```python
from build123d import *

# Parameters (mm, degrees)
SZKIC1_R                    = 4.5
SZKIC1_R_2                  = 6.5
DODANIE_WYCI_GNI_CIE1_DEPTH = 10


with BuildPart() as part:
    # Szkic1 → Dodanie-wyciągnięcie1 (new body)
    with BuildSketch(Plane(origin=(0, 0, 0), x_dir=(1, 0, 0), z_dir=(0, 1, 0))):
        with BuildLine():
            Line((-1.5, 30.463092423), (-1.5, 29.063092423))
            ThreePointArc((-1.5, 29.063092423), (0, 27.563092423), (1.5, 29.063092423))
            Line((1.5, 29.063092423), (1.5, 30.463092423))
            ThreePointArc((1.5, 30.463092423), (0, -30.5), (-1.5, 30.463092423))
        make_face()
        with Locations(Location((0, 0, 0), (0, 0, 270))):
            Circle(SZKIC1_R, mode=Mode.SUBTRACT)
        with Locations(Location((0, 17.5, 0), (0, 0, 270))):
            Circle(SZKIC1_R_2, mode=Mode.SUBTRACT)
        with Locations(Location((13.682050943, 10.911071533, 0), (0, 0, 270))):
            Circle(SZKIC1_R_2, mode=Mode.SUBTRACT)
        with Locations(Location((17.061238463, -3.894116344, 0), (0, 0, 270))):
            Circle(SZKIC1_R_2, mode=Mode.SUBTRACT)
        with Locations(Location((7.592965435, -15.766955188, 0), (0, 0, 270))):
            Circle(SZKIC1_R_2, mode=Mode.SUBTRACT)
        with Locations(Location((-7.592965435, -15.766955188, 0), (0, 0, 270))):
            Circle(SZKIC1_R_2, mode=Mode.SUBTRACT)
        with Locations(Location((-17.061238463, -3.894116344, 0), (0, 0, 270))):
            Circle(SZKIC1_R_2, mode=Mode.SUBTRACT)
        with Locations(Location((-13.682050943, 10.911071533, 0), (0, 0, 270))):
            Circle(SZKIC1_R_2, mode=Mode.SUBTRACT)
    extrude(amount=DODANIE_WYCI_GNI_CIE1_DEPTH)


solid = part.part
```
Design review of the part built by this model. Coordinates are the model's own, in mm. A direction names the side the tool comes from. Give positions to 0.01 mm unless a question says otherwise; leave off trailing zeros. Write each loop counter-clockwise with the first axis right and the second up, starting at its lowest first coordinate (ties: lowest second). Pieces come first, ordered by that corner, then holes.
(1) Mouldability with a two-part tool opening along X and no side actions: class faces 3 (the face through (-6, 10, 0)), 4 (the face through (-13.396, 4.93, -17.405)), 5 (the face through (1.32, 4.93, 30.47)), 6 (the face through (-0.033, 4.93, -27.563)) as +X half, -X half, draft (parallel to the pull), parting line (faces both ways), or undercut.
Checked values:
face 3: draft
face 4: undercut
face 5: parting line
face 6: undercut
(2) Add section A-A (x = 0). Give the boundary of the cut face in (y, z).
Checked values:
outline: (0, -27.56) - (10, -27.56) - (10, -24) - (0, -24) - close; (0, -11) - (10, -11) - (10, -4.5) - (0, -4.5) - close; (0, 4.5) - (10, 4.5) - (10, 30.5) - (0, 30.5) - close
(3) Tool access review of faces 1 (the face through (13.106, 4.93, -1.264)), 2 (the face through (1.5, 5, -30)): name each direction out of +Z, -Z, +X, -X, +Y, -Y from which nothing blocks a thin tool from reaching the whole face with its end or side.
Checked values:
face 1: +Y, -Y
face 2: -Z, +Y, -Y
(4) Wall thickness on line 1 along Z through (x, y) = (-12, 3.75); line 2 along Z through (x, y) = (-10.5, 8); line 3 along X through (y, z) = (8.75, -2): over which ranges is each line inside the solid? List them lowest first.
Checked values:
line 1: z = -28.04 to -17.19, -4.63 to -0.18, 7.97 to 10.99, 20.54 to 28.04
line 2: z = -28.64 to -16.58, -5.24 to 9.95, 21.58 to 28.64
line 3: x = -30.43 to -19.8, -14.32 to -4.03, 4.03 to 14.32, 19.8 to 30.43
(5) Clearance check with flat-ended pins moving along their axes: pin 1 Ø2 at (x, z) = (2, 2.5) entering from +Y; pin 2 Ø3 at (x, y) = (13, 7) entering from +Z. State where each tip first meets the part, or that it passes through.
Checked values:
pin 1: passes through
pin 2: stops at z = 28.25
(6) Add section D-D (y = 6.25). Give the number of separate pieces and of enclosed holes in the cut face, and give its area (3 significant figures).
Checked values:
separate pieces: 1
enclosed holes: 8
area: 1,920 mm2
(7) Add section C-C (z = 11.5). Give the boundary of the cut face in (x, y).
Checked values:
outline: (-28.25, 0) - (-12.5, 0) - (-12.5, 10) - (-28.25, 10) - close; (-2.69, 0) - (2.69, 0) - (2.69, 10) - (-2.69, 10) - close; (12.5, 0) - (28.25, 0) - (28.25, 10) - (12.5, 10) - close
(8) Add section B-B (z = -22). Give the boundary of the cut face in (x, y), and give its area (3 significant figures).
Checked values:
outline: (-21.12, 0) - (-4.69, 0) - (-4.69, 10) - (-21.12, 10) - close; (4.69, 0) - (21.12, 0) - (21.12, 10) - (4.69, 10) - close
area: 329 mm2
